For this review, use the dimensioned drawing (mm, ordinates from the lowest corner) and the shaded views. A direction names the side the tool comes from. Coordinates: 2 decimals unless noted, no trailing zeros. Order: outer loops, then holes, each group sorted by start corner. A loop starts at its lowest first (then second) coordinate and runs counter-clockwise, first axis right, second up. Notation, with made-up numbers: M -21.5,20 L 19.5,20 A21 ccw 19.5,49 Z; hole C -33.75,71.5 d7. An arc over 180 degrees is marked long. Answer in a Markdown table with one row per item.
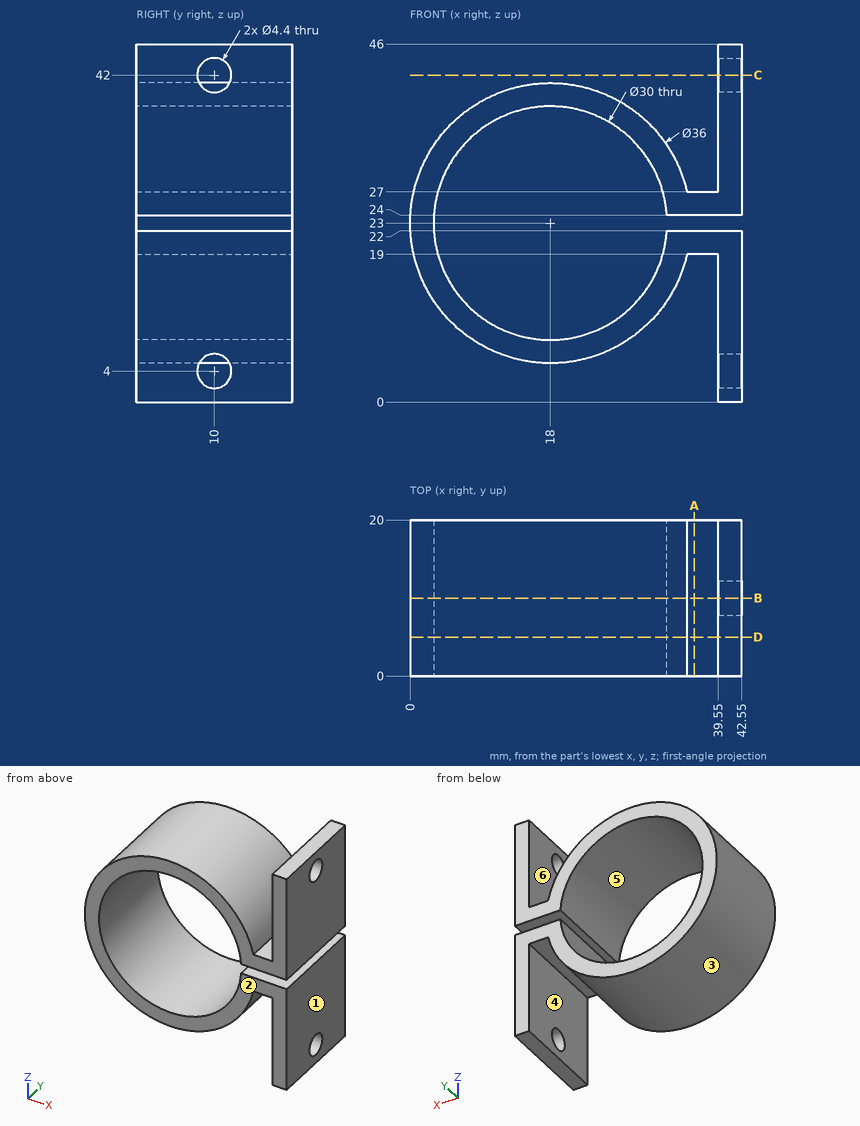
(1) Machinability: for the marked faces 4, 5 and 6, which of the approach directions +Z, -Z, +X, -X, +Y, -Y give a long, thin tool a straight path to every point of the face, cutting with its end or side? Answer none if there is none.
Report:
| item | result |
|---|---|
| face 4 | -Z, +Y, -Y |
| face 5 | +Y, -Y |
| face 6 | +Z, +Y, -Y |
(2) Take a section at D-D (y = 5). Write out the cut boundary in (x, z).
Report:
| item | result |
|---|---|
| outline | M 32.97,22 A15 cw long 32.97,24 L 42.55,24 L 42.55,46 L 39.55,46 L 39.55,27 L 35.55,27 A18 ccw long 35.55,19 L 39.55,19 L 39.55,0 L 42.55,0 L 42.55,22 Z |
(3) To check wall thickness, follow line 1 (Y direction, x = 40.65, z = 4); line 2 (Z direction, x = 39, y = 10.25); line 3 (Z direction, x = 18.5, y = 3.5). State the ranges of each line that lie inside material, in increasing order. Write a range as [from, to].
Report:
| item | result |
|---|---|
| line 1 | [0, 7.8], [12.2, 20] |
| line 2 | [19, 22], [24, 27] |
| line 3 | [5.01, 8.01], [37.99, 40.99] |
(4) Take a section at B-B (y = 10). Write out the cut boundary in (x, z), then the cut area to 3 significant figures.
Report:
| item | result |
|---|---|
| outline | M 32.97,22 A15 cw long 32.97,24 L 42.55,24 L 42.55,39.8 L 39.55,39.8 L 39.55,27 L 35.55,27 A18 ccw long 35.55,19 L 39.55,19 L 39.55,6.2 L 42.55,6.2 L 42.55,22 Z; M 39.55,0 L 42.55,0 L 42.55,1.8 L 39.55,1.8 Z; M 39.55,44.2 L 42.55,44.2 L 42.55,46 L 39.55,46 Z |
| area | 433 mm^2 |
(5) Insertion check: P1, Ø9.5, axis at y = 12, z = 37, coming from the -X side; P2, Ø1.2, axis at x = 38, y = 6, coming from the +Z side; P3, Ø4.5, axis at x = 38.5, y = 7.5, coming from the -Z side; P4, Ø5, axis at x = 27, y = 11.5, coming from the +Z side. Each pin has a flat end and moves straight along its axis. Give the tip position at first contact, or say it passes through.
Report:
| item | result |
|---|---|
| P1 | x = 2.56 |
| P2 | z = 27 |
| P3 | z = 0 |
| P4 | z = 39.79 |
(6) The part is to be moulded in two halves that separate along X. For the marked faces 1, 2 and 3, say which applies: +X half, -X half, draft (parallel to the pull), parting line (faces both ways), or undercut.
Report:
| item | result |
|---|---|
| face 1 | +X half |
| face 2 | draft |
| face 3 | undercut |
(7) Take a section at C-C (z = 42). Write out the cut boundary in (x, y).
Report:
| item | result |
|---|---|
| outline | M 39.55,0 L 42.55,0 L 42.55,7.8 L 39.55,7.8 Z; M 39.55,12.2 L 42.55,12.2 L 42.55,20 L 39.55,20 Z |
(8) Take a section at A-A (x = 36.5). Write out the cut boundary in (y, z), then the cut area to 3 significant figures.
Report:
| item | result |
|---|---|
| outline | M 0,19 L 20,19 L 20,22 L 0,22 Z; M 0,24 L 20,24 L 20,27 L 0,27 Z |
| area | 120 mm^2 |
